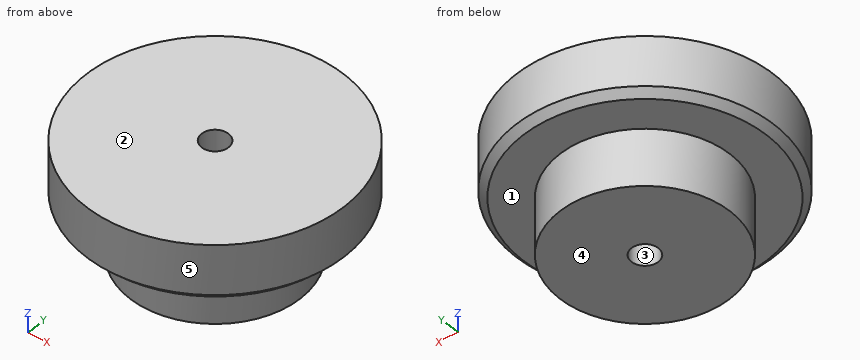
from build123d import *

# Parameters (mm, degrees)
F3_D     = 2.0574
F5_D     = 3
F5_DEPTH = 19.05
F5_TIP   = 0.9012909285
F6_SIZE  = 0.79375


with BuildPart() as f1:
    # F0 (on Front) → F1 (revolve)
    with BuildSketch(Plane.XZ):
        Polygon((14.4272, 0), (0, 0), (0, -12.7), (9.525, -12.7), (9.525, -6.35), (14.4272, -6.35), align=None)
    revolve(axis=Axis((0, 0, -6.35), (0, 0, 1)))

    # F3 (through all)
    with Locations(Plane.XY):
        with Locations((0, 0)):
            Hole(F3_D / 2)

    # F5
    with Locations(Plane(origin=(0, 0, -12.7), x_dir=(1, 0, 0), z_dir=(0, 0, -1))):
        with Locations((0, 0)):
            Hole(F5_D / 2, depth=F5_DEPTH)
            with Locations((0, 0, -(F5_DEPTH + F5_TIP / 2))):  # 118° drill point
                Cone(0, F5_D / 2, F5_TIP, mode=Mode.SUBTRACT)

    # F6
    f6_edges = [f1.edges().sort_by_distance(p)[0] for p in [
        (-14.4272, 0, -6.35),
    ]]
    chamfer(f6_edges, length=F6_SIZE)


solid = f1.part
Geometry check sheet. Reference: the model listing, model coordinates, mm. Face numbers are marked on the shaded views. A direction names the side the tool comes from. Round coordinates to 2 decimals unless told otherwise and drop trailing zeros. Loops run counter-clockwise (first coordinate to the right, second up) from the corner with the lowest first, then second, coordinate; pieces in that order, holes last.
Item 1: Gauge pin test, flat ends, axial feed: pin 1 (2 mm diameter, centred on x = 7, y = -10.5, fed in from -Z); pin 2 (2.5 mm diameter, centred on x = 0, y = 0, fed in from -Z); pin 3 (4 mm diameter, centred on y = -8, z = -8.5, fed in from -X); pin 4 (5 mm diameter, centred on y = 3.5, z = -8.5, fed in from +X). Record the tip position at first contact, or that the pin passes through.
Item 2: Access from +Z, -Z, +X, -X, +Y, -Y to the whole of each face (thin tool, end or side, straight path). Record for the marked faces 1 and 2.
Item 3: Cross-section at A-A on y = 0. Record the boundary of the cut face in (x, z) (3 decimals).
Item 4: Thickness scan on line 1 (Y direction, x = 0, z = -5.5); line 2 (Y direction, x = 0, z = -7.75) (3 decimals); line 3 (Z direction, x = 3.25, y = 9.75). Record the ranges inside material, lowest first.
Item 5: Cross-section at C-C on z = -9.5. Record the boundary of the cut face in (x, y) (3 decimals), then the cut area to 3 significant figures.
Item 6: Mould release check, pull along X, two halves, no side actions. Record for the marked faces 3, 4 and 5: pulls with the +X half, pulls with the -X half, needs draft (parallel to the pull), parting line crosses it, or undercut.
Answer sheet:
1. pin 1: stops at z = -6.35
1. pin 2: passes through
1. pin 3: stops at x = -7.4
1. pin 4: stops at x = 13.61
2. face 1: -Z
2. face 2: +Z, +X, -X, +Y, -Y
3. outline: (-14.427, -5.556) - (-13.633, -6.35) - (-9.525, -6.35) - (-9.525, -12.7) - (-1.5, -12.7) - (-1.5, 0) - (-14.427, 0) - close; (1.5, -12.7) - (9.525, -12.7) - (9.525, -6.35) - (13.633, -6.35) - (14.427, -5.556) - (14.427, 0) - (1.5, 0) - close
4. line 1: y = -14.43 to -1.5, 1.5 to 14.43
4. line 2: y = -9.525 to -1.5, 1.5 to 9.525
4. line 3: z = -6.35 to 0
5. outline: circle Ø19.05 at (0, 0); hole circle Ø3 at (0, 0)
5. area: 278 mm2
6. face 3: undercut
6. face 4: needs draft
6. face 5: parting line crosses it
